The model under review builds one solid part; all positions refer to its coordinate system, in mm. A direction names the side the tool comes from. Round coordinates to 2 decimals unless told otherwise and drop trailing zeros. Write each loop counter-clockwise with the first axis right and the second up, starting at its lowest first coordinate (ties: lowest second). Pieces come first, ordered by that corner, then holes. Notation, with made-up numbers: (-2.75, -23.75) - (29.25, -23.75) arc R19 ccw to (29.25, -3.75) - close; hole circle Ø6 at (26, 74.5). An arc over 180 degrees is marked (long way). Write each question's results on one line, items separated by ' | '.
```python
from build123d import *

# Parameters (mm, degrees)
SKETCH1_W           = 63.5
SKETCH1_H           = 19.05
BOSS_EXTRUDE1_DEPTH = 38.1
SKETCH2_W           = 57.15
SKETCH2_H           = 56.546509541
CUT_EXTRUDE1_DEPTH  = 9.525
BOSS_EXTRUDE3_DEPTH = 19.05
SKETCH6_W           = 31.75
SKETCH6_H           = 41.275
CUT_EXTRUDE3_DEPTH  = 19.05


with BuildPart() as part:
    # Sketch1 → Boss-Extrude1 (new body, symmetric)
    with BuildSketch(Plane(origin=(0, 0, 0), x_dir=(0, 0, -1), z_dir=(1, 0, 0))):
        with Locations((19.525170068, 1.123129252)):
            Rectangle(SKETCH1_W, SKETCH1_H)
    extrude(amount=BOSS_EXTRUDE1_DEPTH, both=True)

    # Sketch2 → Cut-Extrude1 (cut)
    with BuildSketch(Plane(origin=(0, 10.648129252, 0), x_dir=(1, 0, 0), z_dir=(0, 1, 0))):
        with Locations((0, 16.048424839)):
            Rectangle(SKETCH2_W, SKETCH2_H)
    extrude(amount=-CUT_EXTRUDE1_DEPTH, mode=Mode.SUBTRACT)

    # Sketch5 → Boss-Extrude3 (add)
    with BuildSketch(Plane.XZ.offset(8.401870748)):
        Polygon((-25.4, 12.224829932), (-15.875, 12.224829932), (-15.875, -29.050170068), (15.875, -29.050170068), (15.875, 12.224829932), (25.4, 12.224829932), (25.4, -38.575170068), (-25.4, -38.575170068), align=None)
    extrude(amount=BOSS_EXTRUDE3_DEPTH)

    # Sketch6 → Cut-Extrude3 (cut)
    with BuildSketch(Plane.XZ.offset(8.401870748)):
        with Locations((0, -8.412670068)):
            Rectangle(SKETCH6_W, SKETCH6_H)
    extrude(amount=-CUT_EXTRUDE3_DEPTH, mode=Mode.SUBTRACT)


solid = part.part
```
Q1. We need section C-C (x = -10). State the section outline as (y, z) points.
Evaluation:
outline: (-27.45, -38.58) - (-8.4, -38.58) - (-8.4, -51.28) - (10.65, -51.28) - (10.65, -44.32) - (1.12, -44.32) - (1.12, -29.05) - (-27.45, -29.05) - close
Q2. We need section B-B (y = 4). State the section outline as (x, z) points (3 decimals).
Evaluation:
outline: (-38.1, -51.275) - (38.1, -51.275) - (38.1, 12.225) - (28.575, 12.225) - (28.575, -44.322) - (-28.575, -44.322) - (-28.575, 12.225) - (-38.1, 12.225) - close
Q3. We need section D-D (x = 27.5). State the section outline as (y, z) points, plus the area to 3 significant figures.
Evaluation:
outline: (-8.4, -51.28) - (10.65, -51.28) - (10.65, -44.32) - (1.12, -44.32) - (1.12, 12.22) - (-8.4, 12.22) - close | area: 671 mm^2
Q4. For probe 1 along X at (y, z) = (7.5, -25) (3 decimals); probe 2 along X at (y, z) = (-26, 7) (3 decimals); probe 3 along Z at (x, y) = (16.5, 5), list the stretches that pass through material, from the lowest coordinate up.
Evaluation:
probe 1: x = -38.1 to -28.575, 28.575 to 38.1 | probe 2: x = -25.4 to -15.875, 15.875 to 25.4 | probe 3: z = -51.28 to -44.32
Q5. Tool access review of faces 1 (the flat face through (0, 1.123, -35)), 2 (the flat face through (0, -13, -29.05)), 3 (the flat face through (0, -18, -38.575)), 4 (the flat face through (25.4, -18, -13)): name each direction out of +Z, -Z, +X, -X, +Y, -Y from which nothing blocks a thin tool from reaching the whole face with its end or side.
Evaluation:
face 1: +Z, +Y | face 2: +Z, +Y, -Y | face 3: -Z, +X, -X, -Y | face 4: +Z, -Z, +X, -Y
Q6. Insertion check: P1, Ø3, axis at x = 3.5, y = 7, coming from the +Z side; P2, Ø21, axis at x = 0.5, y = -16, coming from the -Z side; P3, Ø9.5, axis at y = -17, z = -10, coming from the -X side; P4, Ø17, axis at x = 4, z = -25, coming from the +Y side. Each pin has a flat end and moves straight along its axis. Give the tip position at first contact, or say it passes through.
Evaluation:
P1: stops at z = -44.32 | P2: stops at z = -51.28 | P3: stops at x = -25.4 | P4: stops at y = 1.12
Q7. We need section A-A (z = -26). State the section outline as (x, y) points (3 decimals).
Evaluation:
outline: (-38.1, -8.402) - (-25.4, -8.402) - (-25.4, -27.452) - (-15.875, -27.452) - (-15.875, 1.123) - (-28.575, 1.123) - (-28.575, 10.648) - (-38.1, 10.648) - close; (15.875, -27.452) - (25.4, -27.452) - (25.4, -8.402) - (38.1, -8.402) - (38.1, 10.648) - (28.575, 10.648) - (28.575, 1.123) - (15.875, 1.123) - close
